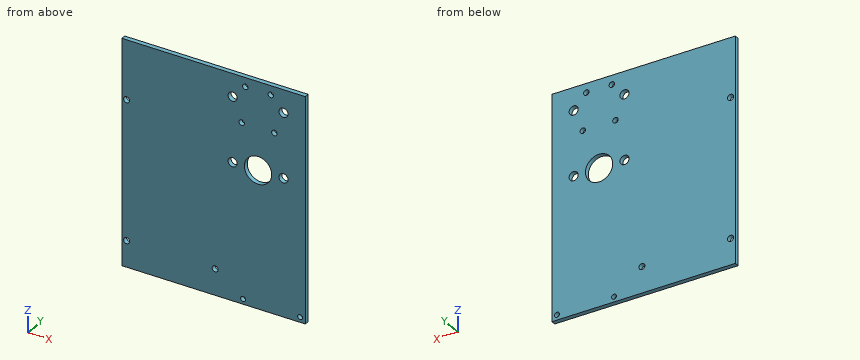
Autodesk Inventor part; units mm, degrees
ref_plane "Work Plane1" through (0, 0, 48) normal (1, 0, 0) x (0, 0, -1)
ref_plane "YZ Plane" through (0, 0, 0) normal (1, 0, 0) x (0, 1, 0)
ref_plane "XZ Plane" through (0, 0, 0) normal (0, 1, 0) x (-1, 0, 0)
sketch "Sketch1" plane through (0, 0, 0) normal (0, 1, 0) x (-1, 0, 0)
  line L0 (75, 48) -> (75, -75)
  line L1 (75, -75) -> (-26, -75)
  line L2 (-26, -75) -> (-26, 48)
  line L3 (75, 48) -> (-26, 48)
  point P0 (0, 0)
extrude "Extrusion1" add sketch "Sketch1" along normal blind 2.5
sketch "Sketch2" plane through (0, 2.5, 0) normal (0, 1, 0) x (1, 0, 0)
  circle A0 centre (0, 0) radius 7.5
  dimension "d4" = 15
extrude "Extrusion2" cut sketch "Sketch2" against normal blind 2.5
ref_plane "Work Plane1" through (0, 0, 48) normal (1, 0, 0) x (0, 0, -1)
sketch "Sketch3" plane through (0, 0, 0) normal (0, -1, 0) x (1, 0, 0)
  circle A0 centre (7, 43) radius 1.5
  line L0 (26, 48) -> (26, -75)
  line L1 (-75, 48) -> (26, 48)
  circle A1 centre (9, 23) radius 1.5
  point P0 (0, 0)
  dimension "d12" = 3
  dimension "d15" = 19
  dimension "d18" = 3
  dimension "d19" = 17
  dimension "d20" = 25
  dimension "d21" = 5
extrude "Extrusion3" cut sketch "Sketch3" against normal blind 2.5
mirror "Mirror1" about plane through (0, 0, 48) normal (1, 0, 0) of "Extrusion3"
sketch "Sketch4" plane through (0, 0, 0) normal (0, -1, 0) x (1, 0, 0)
  line L0 (-75, 48) -> (26, 48)
  circle A0 centre (14, 35.5) radius 2.5
  circle A1 centre (14, 0) radius 2.5
  point P0 (0, 0)
  dimension "d24" = 5
  dimension "d28" = 5
  dimension "d29" = 14
  dimension "d30" = 14
extrude "Extrusion4" cut sketch "Sketch4" against normal blind 2.5
mirror "Mirror2" about plane through (0, 0, 48) normal (1, 0, 0) of "Extrusion4"
sketch "Sketch5" plane through (0, 0, 0) normal (0, -1, 0) x (1, 0, 0)
  line L0 (26, 48) -> (26, -75)
  circle A0 centre (23.15, -72.15) radius 1.35
  point P0 (0, 0)
  dimension "d33" = 2.7
extrude "Extrusion5" cut sketch "Sketch5" against normal blind 2.5
pattern_linear "Rectangular Pattern1" count 2 spacing 31.4 along (-1, 0, 0) of "Extrusion5"
sketch "Sketch6" plane through (0, 0, 0) normal (0, -1, 0) x (1, 0, 0)
  circle A0 centre (-72.4, -60.65) radius 1.65
  point P0 (0, 0)
  point P1 (-75, -75)
  dimension "d41" = 3.3
extrude "Extrusion6" cut sketch "Sketch6" against normal blind 2.5
pattern_linear "Rectangular Pattern2" count 2 spacing 48.8 along (1, 0, 0) of "Extrusion6"
pattern_linear "Rectangular Pattern3" count 2 spacing 76.25 along (0, 0, 1) of "Extrusion6"
properties part number "BaseMDF"
Geometry check sheet. Reference: the model listing, model coordinates, mm. Give positions to 0.01 mm unless a question says otherwise; leave off trailing zeros. Write each loop counter-clockwise with the first axis right and the second up, starting at its lowest first coordinate (ties: lowest second). Pieces come first, ordered by that corner, then holes. Notation, with made-up numbers: M 66.5,-22 L 120.5,-22 A18 cw 120.5,-17 Z; hole C 73,36.25 d6. An arc over 180 degrees is marked long. Answer as CSV lines item,"result". Start each with the question number.
Q1. Go/stop test with a flat-tipped pin: pin 1 (13.5 mm diameter, centred on x = 0, z = 0, fed in from +Y) (3 decimals). Record where the tip stops, or that it passes through.
Q2. Section check A-A, the plane x = -14. Record the cut outline in (y, z), then the cut area to 4 significant figures.
Q3. Material ranges on L1, parallel to X at y = 0.9, z = -72.15; L2, parallel to Z at x = 0, y = 1.55; L3, parallel to Z at x = 14, y = 0.7, recorded low to high.
Q4. Section check B-B, the plane z = 35.5. Record the cut outline in (x, y), then the cut area to 4 significant figures.
Q5. Section check D-D, the plane y = 1.6. Give the number of separate pieces and of enclosed holes in the cut face, then the cut area to 3 significant figures.
Q6. Section check C-C, the plane x = 0. Record the cut outline in (y, z).
Geometry says:
1,pin 1,"through"
2,outline,"M 0,-75 L 2.5,-75 L 2.5,-2.5 L 0,-2.5 Z; M 0,2.5 L 2.5,2.5 L 2.5,33 L 0,33 Z; M 0,38 L 2.5,38 L 2.5,48 L 0,48 Z"
2,area,"282.5 mm^2"
3,L1,"-75 to -9.6, -6.9 to 21.8, 24.5 to 26"
3,L2,"-75 to -7.5, 7.5 to 48"
3,L3,"-75 to -2.5, 2.5 to 33, 38 to 48"
4,outline,"M -75,0 L -16.5,0 L -16.5,2.5 L -75,2.5 Z; M -11.5,0 L 11.5,0 L 11.5,2.5 L -11.5,2.5 Z; M 16.5,0 L 26,0 L 26,2.5 L 16.5,2.5 Z"
4,area,"227.5 mm^2"
5,separate pieces,"1"
5,enclosed holes,"14"
5,area,"12,100 mm^2"
6,outline,"M 0,-75 L 2.5,-75 L 2.5,-7.5 L 0,-7.5 Z; M 0,7.5 L 2.5,7.5 L 2.5,48 L 0,48 Z"
